```python
from build123d import *

# Parameters (mm, degrees)
BASE_FLANGE1_DEPTH = 10
SKETCH6_R          = 2.5
CUT_EXTRUDE1_DEPTH = 35.932076949
SKETCH7_R          = 2
CUT_EXTRUDE2_DEPTH = 36.305806888
FILLET1_R          = 2


# Sheet-metal steps are written as plain solids
with BuildPart() as part:
    # Sketch1 → Base-Flange1 (new body)
    with BuildSketch(Plane.XY):
        with BuildLine():
            Line((0, 0), (13, 0))
            ThreePointArc((13, 0), (13.530330086, 0.219669914), (13.75, 0.75))
            Line((13.75, 0.75), (13.75, 5.75))
            ThreePointArc((13.75, 5.75), (14.409009742, 7.340990258), (16, 8))
            Line((16, 8), (32.5, 8))
            Line((32.5, 8), (32.5, 6.5))
            Line((32.5, 6.5), (16, 6.5))
            ThreePointArc((16, 6.5), (15.469669914, 6.280330086), (15.25, 5.75))
            Line((15.25, 5.75), (15.25, 0.75))
            ThreePointArc((15.25, 0.75), (14.590990258, -0.840990258), (13, -1.5))
            Line((13, -1.5), (0, -1.5))
            Line((0, -1.5), (0, 0))
        make_face()
    extrude(amount=BASE_FLANGE1_DEPTH)

    # Sketch6 → Cut-Extrude1 (cut, through all)
    with BuildSketch(Plane(origin=(0, 0, 0), x_dir=(1, 0, 0), z_dir=(0, 1, 0))):
        with Locations(Location((7.5, -5, 0), (0, 0, 270))):
            Circle(SKETCH6_R)
    extrude(amount=-CUT_EXTRUDE1_DEPTH, mode=Mode.SUBTRACT)

    # Sketch7 → Cut-Extrude2 (cut, through all)
    with BuildSketch(Plane(origin=(0, 8, 0), x_dir=(1, 0, 0), z_dir=(0, 1, 0))):
        with Locations(Location((27.5, -5, 0), (0, 0, 270))):
            Circle(SKETCH7_R)
    extrude(amount=-CUT_EXTRUDE2_DEPTH, mode=Mode.SUBTRACT)

    # Fillet1
    fillet1_edges = [part.edges().sort_by_distance(p)[0] for p in [
        (0, -0.75, 0),
        (32.5, 7.25, 0),
        (0, -0.75, 10),
        (32.5, 7.25, 10),
    ]]
    fillet(fillet1_edges, radius=FILLET1_R)


solid = part.part
```
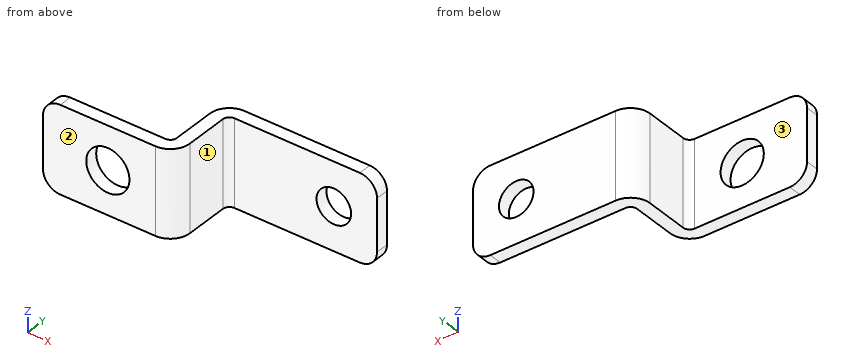
The listing builds one solid part. Answer for the finished solid, in the listing's coordinates (mm). Face numbers are marked on the shaded views. A direction names the side the tool comes from. Give positions to 0.01 mm unless a question says otherwise; leave off trailing zeros. Write each loop counter-clockwise with the first axis right and the second up, starting at its lowest first coordinate (ties: lowest second). Pieces come first, ordered by that corner, then holes. Notation, with made-up numbers: (33, 20) -> (53, 20) arc R26 ccw to (53, 34) -> close; hole circle Ø2 at (85, 42). An arc over 180 degrees is marked (long way). Use one line per item in the form item = value.
1) Each of these flat-tipped pins is pushed along its axis until it touches: P1, Ø5, axis at y = 4, z = 4.5, coming from the -X side; P2, Ø3, axis at x = 7, z = 5.5, coming from the +Y side; P3, Ø1.5, axis at x = 14.5, y = 1.5, coming from the -Z side; P4, Ø1.5, axis at y = 4, z = 6, coming from the +X side. Where does it stop, or does it pass through?
Result:
P1 = 13.75
P2 = through
P3 = 0
P4 = 15.25
2) Section D-D on z = 9.25 is taken. Write down the section's boundary in (x, y).
Result:
outline = (0.44, -1.5) -> (13, -1.5) arc R2.25 ccw to (15.25, 0.75) -> (15.25, 5.75) arc R0.75 cw to (16, 6.5) -> (32.06, 6.5) -> (32.06, 8) -> (16, 8) arc R2.25 ccw to (13.75, 5.75) -> (13.75, 0.75) arc R0.75 cw to (13, 0) -> (0.44, 0) -> close
3) Section B-B on x = 7.5 is taken. Write down the section's boundary in (y, z), plus the area to 3 significant figures.
Result:
outline = (-1.5, 0) -> (0, 0) -> (0, 2.5) -> (-1.5, 2.5) -> close; (-1.5, 7.5) -> (0, 7.5) -> (0, 10) -> (-1.5, 10) -> close
area = 7.50 mm²
4) Straight lines are drawn through the part: probe 1 along X at (y, z) = (2.75, 5.5); probe 2 along X at (y, z) = (-0.7, 5); probe 3 along X at (y, z) = (-0.95, 5). For each, find the intervals that lie inside material, in ascending order.
Result:
probe_1 = 13.75 to 15.25
probe_2 = 0 to 5, 10 to 14.72
probe_3 = 0 to 5, 10 to 14.47
5) A tool of negligible diameter and unlimited length cuts with its end or side. For the marked faces 1, 2 and 3, from which of +Z, -Z, +X, -X, +Y, -Y can it reach the whole face along a straight path? Write none if from no direction.
Result:
face_1 = +Z, -Z, +X, -Y
face_2 = +Z, -Z, +X, -X, -Y
face_3 = +Z, -Z, -X, +Y
6) Section A-A on z = 5 is taken. Write down the section's boundary in (x, y), plus the area to 3 significant figures.
Result:
outline = (0, -1.5) -> (5, -1.5) -> (5, 0) -> (0, 0) -> close; (10, -1.5) -> (13, -1.5) arc R2.25 ccw to (15.25, 0.75) -> (15.25, 5.75) arc R0.75 cw to (16, 6.5) -> (25.5, 6.5) -> (25.5, 8) -> (16, 8) arc R2.25 ccw to (13.75, 5.75) -> (13.75, 0.75) arc R0.75 cw to (13, 0) -> (10, 0) -> close; (29.5, 6.5) -> (32.5, 6.5) -> (32.5, 8) -> (29.5, 8) -> close
area = 45.3 mm²
7) Section C-C on y = -0.5 is taken. Write down the section's boundary in (x, z), plus the area to 3 significant figures.
Result:
outline = (0, 2) arc R2 ccw to (2, 0) -> (14.87, 0) -> (14.87, 10) -> (2, 10) arc R2 ccw to (0, 8) -> close; hole circle Ø5 at (7.5, 5)
area = 127 mm²
